The figure shows three views and two pictorial views of one solid part (mm, origin at its lowest corner). Answer the questions. A direction names the side the tool comes from. Give positions to 0.01 mm unless a question says otherwise; leave off trailing zeros. Write each loop counter-clockwise with the first axis right and the second up, starting at its lowest first coordinate (ties: lowest second). Pieces come first, ordered by that corner, then holes. Notation, with made-up numbers: M 40.25,23 L 44.25,23 A22 cw 44.25,31 Z; hole C -6.75,21 d3. An arc over 180 degrees is marked long. Return JSON: item names as keys, results as strings.
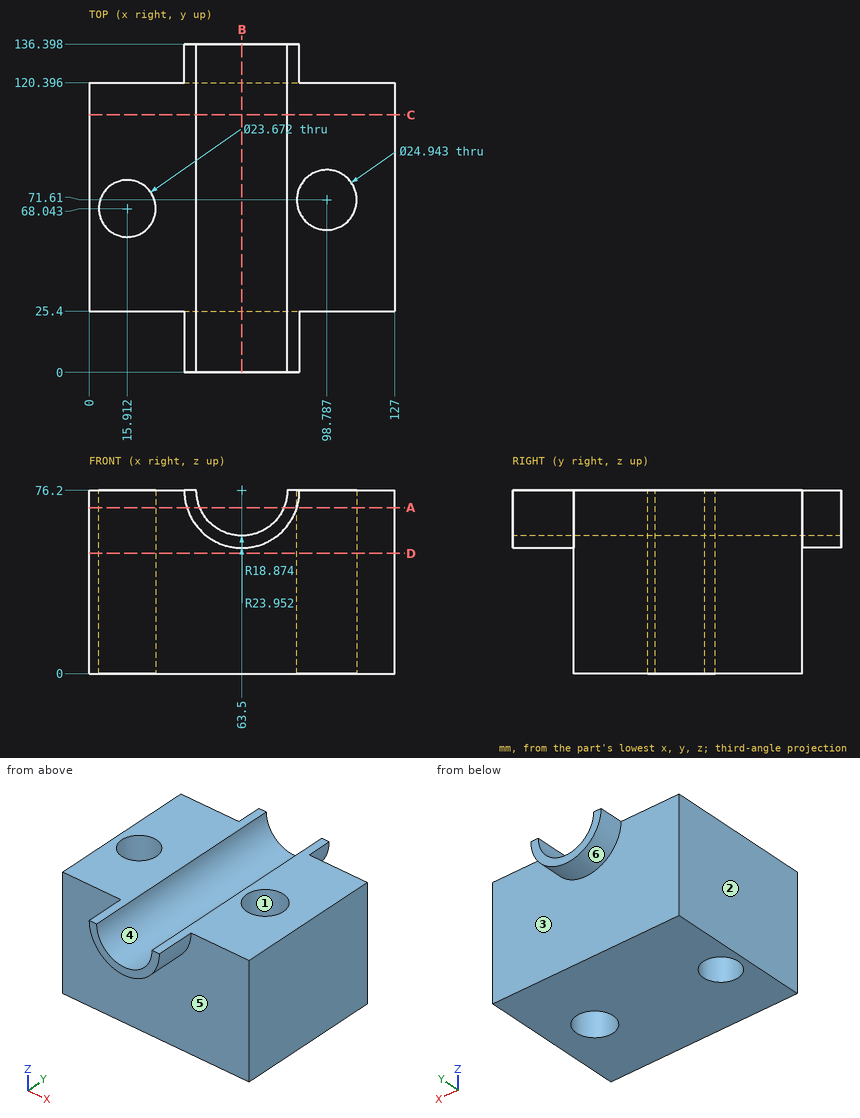
Item 1: Determine the mould class of the marked faces 1, 2 and 3 for opening direction Y: +Y half, -Y half, draft (parallel to the pull), parting line (faces both ways), or undercut.
Geometry results:
{"face 1": "undercut", "face 2": "draft", "face 3": "+Y half"}
Item 2: A cutting plane is placed at A-A, the plane z = 69. Write down the section's boundary in (x, y) (1 decimal), plus the area to 3 significant figures.
Geometry results:
{"outline": "M 0,25.4 L 40.7,25.4 L 40.7,0 L 46.1,0 L 46.1,136.4 L 40.7,136.4 L 40.7,120.4 L 0,120.4 Z; M 80.9,0 L 86.3,0 L 86.3,25.4 L 127,25.4 L 127,120.4 L 86.3,120.4 L 86.3,136.4 L 80.9,136.4 Z; hole C 15.9,68 d23.7; hole C 98.8,71.6 d24.9", "area": "8,270 mm2"}
Item 3: A cutting plane is placed at B-B, the plane x = 63.5. Write down the section's boundary in (y, z), plus the area to 3 significant figures.
Geometry results:
{"outline": "M 0,52.25 L 25.4,52.25 L 25.4,0 L 120.4,0 L 120.4,52.25 L 136.4,52.25 L 136.4,57.33 L 0,57.33 Z", "area": "5,660 mm2"}
Item 4: A cutting plane is placed at D-D, the plane z = 50. Write down the section's boundary in (x, y), plus the area to 3 significant figures.
Geometry results:
{"outline": "M 0,25.4 L 127,25.4 L 127,120.4 L 0,120.4 Z; hole C 15.91,68.04 d23.67; hole C 98.79,71.61 d24.94", "area": "11,100 mm2"}
Item 5: A cutting plane is placed at C-C, the plane y = 107. Write down the section's boundary in (x, z).
Geometry results:
{"outline": "M 0,0 L 127,0 L 127,76.2 L 82.37,76.2 A18.87 cw 44.63,76.2 L 0,76.2 Z"}
Item 6: Given pin 1 Ø2 at (x, z) = (39, 53) entering from -Y; pin 2 Ø23 at (x, z) = (95, 54.5) entering from +Y, each flat-ended and moving along its own axis, determine where each tip first touches the part or whether it passes through.
Geometry results:
{"pin 1": "stops at y = 25.4", "pin 2": "stops at y = 120.4"}
Item 7: Which of the six approach directions +Z, -Z, +X, -X, +Y, -Y give full straight-line access (tool end or side, diameter ignored) to the marked faces 4, 5 and 6?
Geometry results:
{"face 4": "+Z, +Y, -Y", "face 5": "-Z, -Y", "face 6": "-Z, +Y"}
Item 8: Find the intervals of material crossed by line 1 (X direction, y = 69.5, z = 19.5) (1 decimal); line 2 (X direction, y = 61, z = 6) (1 decimal); line 3 (Y direction, x = 86, z = 10), in increasing order.
Geometry results:
{"line 1": "x = 0 to 4.2, 27.7 to 86.5, 111.1 to 127", "line 2": "x = 0 to 6.4, 25.4 to 92.2, 105.3 to 127", "line 3": "y = 25.4 to 120.4"}
